```python
from build123d import *

# Parameters (mm, degrees)
SKETCH1_W                       = 220
SKETCH1_H                       = 217
BLOCO_BRUTO_DEPTH               = 26
SKETCH2_R                       = 8.5
FURO_17_PASSANTE_DEPTH          = 157.678811586
SKETCH2_3_R                     = 17.5
SKETCH2_3_R_2                   = 8.5
REBAIXO_35X20_DEPTH             = 20
SKETCH2_4_R                     = 30
SKETCH2_4_R_2                   = 17.5
REBAIXO_60X10_DEPTH             = 10
REBAIXO_220X81X15_DEPTH         = 15
REBAIXO_ENCAIXE_MANCAIS_DEPTH   = 5
M6X1_0_FUROS_APOIO_D            = 5
M6X1_0_FUROS_APOIO_DEPTH        = 17
M6X1_0_FUROS_APOIO_CSINK_D      = 6.05
M6X1_0_FUROS_APOIO_CSINK_ANGLE  = 90
M6X1_0_FUROS_APOIO_TIP          = 1.502151548
M4X0_7_TAPPED_HOLE1_D           = 3.3
M4X0_7_TAPPED_HOLE1_DEPTH       = 11.5
M4X0_7_TAPPED_HOLE1_CSINK_D     = 4.05
M4X0_7_TAPPED_HOLE1_CSINK_ANGLE = 90
M4X0_7_TAPPED_HOLE1_TIP         = 0.991420021


with BuildPart() as part:
    # Sketch1 → Bloco (Bruto) (new body)
    with BuildSketch(Plane(origin=(0, 0, 0), x_dir=(1, 0, 0), z_dir=(0, 1, 0))):
        Rectangle(SKETCH1_W, SKETCH1_H)
    extrude(amount=BLOCO_BRUTO_DEPTH)

    # Sketch2 → Furo Ø17 Passante (cut, through all)
    with BuildSketch(Plane(origin=(0, 26, 0), x_dir=(1, 0, 0), z_dir=(0, 1, 0))):
        with Locations(Location((0, -8.5, 0), (0, 0, 270))):
            Circle(SKETCH2_R)
    extrude(amount=-FURO_17_PASSANTE_DEPTH, mode=Mode.SUBTRACT)

    # Sketch2<3> → Rebaixo Ø35x20 (cut)
    with BuildSketch(Plane(origin=(0, 26, 0), x_dir=(1, 0, 0), z_dir=(0, 1, 0))):
        with Locations(Location((0, -8.5, 0), (0, 0, 270))):
            Circle(SKETCH2_3_R)
        with Locations(Location((0, -8.5, 0), (0, 0, 270))):
            Circle(SKETCH2_3_R_2, mode=Mode.SUBTRACT)
    extrude(amount=-REBAIXO_35X20_DEPTH, mode=Mode.SUBTRACT)

    # Sketch2<4> → Rebaixo Ø60x10 (cut)
    with BuildSketch(Plane(origin=(0, 26, 0), x_dir=(1, 0, 0), z_dir=(0, 1, 0))):
        with Locations(Location((0, -8.5, 0), (0, 0, 270))):
            Circle(SKETCH2_4_R)
        with Locations(Location((0, -8.5, 0), (0, 0, 270))):
            Circle(SKETCH2_4_R_2, mode=Mode.SUBTRACT)
    extrude(amount=-REBAIXO_60X10_DEPTH, mode=Mode.SUBTRACT)

    # Sketch3 → Rebaixo 220x81x15 (cut)
    with BuildSketch(Plane(origin=(0, 26, 0), x_dir=(1, 0, 0), z_dir=(0, 1, 0))):
        with BuildLine():
            ThreePointArc((18.648056199, 15), (9.874208829, 19.828430948), (0, 21.5))
            Line((0, 21.5), (0, 15))
            Line((0, 15), (18.648056199, 15))
        make_face()
        with BuildLine():
            Line((0, 15), (0, 21.5))
            ThreePointArc((0, 21.5), (-9.874208829, 19.828430948), (-18.648056199, 15))
            Line((-18.648056199, 15), (0, 15))
        make_face()
        with BuildLine():
            Line((110, 36.5), (110, 96))
            Line((110, 96), (0, 96))
            Line((0, 96), (0, 21.5))
            ThreePointArc((0, 21.5), (9.874208829, 19.828430948), (18.648056199, 15))
            Line((18.648056199, 15), (110, 15))
            Line((110, 15), (110, 32.5))
            Line((110, 32.5), (52.3, 32.5))
            Line((52.3, 32.5), (52.3, 36.5))
            Line((52.3, 36.5), (110, 36.5))
        make_face()
        with BuildLine():
            Line((0, 21.5), (0, 96))
            Line((0, 96), (-110, 96))
            Line((-110, 96), (-110, 36.5))
            Line((-110, 36.5), (-52.3, 36.5))
            Line((-52.3, 36.5), (-52.3, 32.5))
            Line((-52.3, 32.5), (-110, 32.5))
            Line((-110, 32.5), (-110, 15))
            Line((-110, 15), (-18.648056199, 15))
            ThreePointArc((-18.648056199, 15), (-9.874208829, 19.828430948), (0, 21.5))
        make_face()
    extrude(amount=-REBAIXO_220X81X15_DEPTH, mode=Mode.SUBTRACT)

    # Sketch4 → Rebaixo - Encaixe Mancais (cut)
    with BuildSketch(Plane(origin=(0, 11, 0), x_dir=(1, 0, 0), z_dir=(0, 1, 0))):
        with BuildLine():
            Line((-110, 86.5), (-55.3, 86.5))
            ThreePointArc((-55.3, 86.5), (-53.178679656, 85.621320344), (-52.3, 83.5))
            Line((-52.3, 83.5), (-52.3, 39.5))
            ThreePointArc((-52.3, 39.5), (-53.178679656, 37.378679656), (-55.3, 36.5))
            Line((-55.3, 36.5), (-110, 36.5))
            Line((-110, 36.5), (-110, 86.5))
        make_face()
        with BuildLine():
            Line((110, 36.5), (55.3, 36.5))
            ThreePointArc((55.3, 36.5), (53.178679656, 37.378679656), (52.3, 39.5))
            Line((52.3, 39.5), (52.3, 83.5))
            ThreePointArc((52.3, 83.5), (53.178679656, 85.621320344), (55.3, 86.5))
            Line((55.3, 86.5), (110, 86.5))
            Line((110, 86.5), (110, 36.5))
        make_face()
    extrude(amount=-REBAIXO_ENCAIXE_MANCAIS_DEPTH, mode=Mode.SUBTRACT)

    # M6x1.0 - Furos Apoio
    with Locations(Plane(origin=(0, 26, 0), x_dir=(1, 0, 0), z_dir=(0, 1, 0))):
        with Locations((-100, -102.25), (0, -102.25), (100, -102.25), (-100, 102.25), (0, 102.25), (100, 102.25)):
            CounterSinkHole(M6X1_0_FUROS_APOIO_D / 2, M6X1_0_FUROS_APOIO_CSINK_D / 2, depth=M6X1_0_FUROS_APOIO_DEPTH, counter_sink_angle=M6X1_0_FUROS_APOIO_CSINK_ANGLE)
            with Locations((0, 0, -(M6X1_0_FUROS_APOIO_DEPTH + M6X1_0_FUROS_APOIO_TIP / 2))):  # 118° drill point
                Cone(0, M6X1_0_FUROS_APOIO_D / 2, M6X1_0_FUROS_APOIO_TIP, mode=Mode.SUBTRACT)

    # M4x0.7 Tapped Hole1
    with Locations(Plane(origin=(0, 6, 0), x_dir=(1, 0, 0), z_dir=(0, 1, 0))):
        with Locations((-80.3, 81.5), (-80.3, 41.5), (80.3, 81.5), (80.3, 41.5)):
            CounterSinkHole(M4X0_7_TAPPED_HOLE1_D / 2, M4X0_7_TAPPED_HOLE1_CSINK_D / 2, depth=M4X0_7_TAPPED_HOLE1_DEPTH, counter_sink_angle=M4X0_7_TAPPED_HOLE1_CSINK_ANGLE)
            with Locations((0, 0, -(M4X0_7_TAPPED_HOLE1_DEPTH + M4X0_7_TAPPED_HOLE1_TIP / 2))):  # 118° drill point
                Cone(0, M4X0_7_TAPPED_HOLE1_D / 2, M4X0_7_TAPPED_HOLE1_TIP, mode=Mode.SUBTRACT)


solid = part.part
```
Geometry check sheet. Reference: the model listing, model coordinates, mm. A direction names the side the tool comes from. Coordinates: 2 decimals unless noted, no trailing zeros. Order: outer loops, then holes, each group sorted by start corner. A loop starts at its lowest first (then second) coordinate and runs counter-clockwise, first axis right, second up.
Item 1: Section check B-B (y = 13.5). Count the separate pieces of the cut face and the enclosed holes in it, plus the area to 3 significant figures.
Item 2: Section check C-C (x = -92). Enter the section's corners in (y, z).
Item 3: Tool access check on faces 4 (the flat face through (82, 6, -62)), 5 (the cylindrical face through (-1.04, 21.07, 38.48)), 6 (the flat face through (82, 19, -32.5)), 7 (the flat face through (-2, 13, -108.5)), 8 (the flat face through (-2, 26, 46)). Record the directions out of +Z, -Z, +X, -X, +Y, -Y that give a thin tool (end or side, any length) a straight path to the whole face; none if there is none.
Item 4: Depth check by flat-ended pin: pin 1 (4 mm diameter, centred on x = -100, z = -102.25, fed in from +Y); pin 2 (2.5 mm diameter, centred on y = 8, z = -68, fed in from +X); pin 3 (4.5 mm diameter, centred on x = 80.3, z = -81.5, fed in from +Y). Enter the tip coordinate at first touch or a pass-through.
Item 5: Section check A-A (z = 8.5). Enter the section's corners in (x, y).
Item 6: Mould release check, pull along X, two halves, no side actions. Record for faces 1 (the flat face through (52.3, 9, -61)), 2 (the flat face through (-81, 16, -36.5)), 3 (the cylindrical face through (100.33, 17.12, -104.73)): released by +X, released by -X, zero draft, split by the parting line, or undercut.
Item 7: Scan lines: line 1 along Z through (x, y) = (100, 15.5); line 2 along X through (y, z) = (18.5, 102.25); line 3 along Z through (x, y) = (-71.5, 21). Record each from-to range of solid material in increasing order.
Check sheet entries:
1. separate pieces: 4
1. enclosed holes: 7
1. area: 29,300 mm2
2. outline: (0, -108.5) - (26, -108.5) - (26, -96) - (11, -96) - (11, -86.5) - (6, -86.5) - (6, -36.5) - (26, -36.5) - (26, -32.5) - (11, -32.5) - (11, -15) - (26, -15) - (26, 108.5) - (0, 108.5) - close
3. face 4: +X, +Y
3. face 5: +Y
3. face 6: +X, -X, +Y
3. face 7: -Z, +X, -X, +Y, -Y
3. face 8: +Z, -Z, +X, -X, +Y
4. pin 1: stops at y = 8.7
4. pin 2: stops at x = 52.3
4. pin 3: stops at y = 6
5. outline: (-110, 0) - (-8.5, 0) - (-8.5, 6) - (-17.5, 6) - (-17.5, 16) - (-30, 16) - (-30, 26) - (-110, 26) - close; (8.5, 0) - (110, 0) - (110, 26) - (30, 26) - (30, 16) - (17.5, 16) - (17.5, 6) - (8.5, 6) - close
6. face 1: released by +X
6. face 2: zero draft
6. face 3: undercut
7. line 1: z = -108.5 to -104.75, -99.75 to -96, -36.5 to -32.5, -15 to 99.75, 104.75 to 108.5
7. line 2: x = -110 to -102.5, -97.5 to -2.5, 2.5 to 97.5, 102.5 to 110
7. line 3: z = -108.5 to -96, -36.5 to -32.5, -15 to 108.5
